```python
from build123d import *

# Parameters (mm, degrees)
SKETCH1_W             = 15
SKETCH1_H             = 15
SKETCH1_R             = 2.6
BOSS_EXTRUDE1_DEPTH   = 6
BOSS_EXTRUDE1_2_DEPTH = 6
BOSS_EXTRUDE1_3_DEPTH = 6
BOSS_EXTRUDE1_4_DEPTH = 6
BOSS_EXTRUDE2_DEPTH   = 64
SKETCH2_R             = 3.05
CUT_EXTRUDE1_DEPTH    = 8
SKETCH3_W             = 15
SKETCH3_H             = 15
SKETCH3_R             = 4.5
BOSS_EXTRUDE3_DEPTH   = 4
CHAMFER1_SIZE         = 0.8
SKETCH4_W             = 200
SKETCH4_H             = 8
BOSS_EXTRUDE4_DEPTH   = 15.5
SKETCH5_W             = 200
SKETCH5_H             = 3
BOSS_EXTRUDE5_DEPTH   = 6
FILLET3_R             = 7.5
FILLET4_R             = 1.5


# Some blends are built 0.0001 mm under size
with BuildPart() as part:
    # Sketch1 → Boss-Extrude1 (new body)
    with BuildSketch(Plane.XY):
        with Locations((-25, 15)):
            Rectangle(SKETCH1_W, SKETCH1_H)
        with Locations((-25, 15)):
            Circle(SKETCH1_R, mode=Mode.SUBTRACT)
    extrude(amount=BOSS_EXTRUDE1_DEPTH)



with BuildPart() as body_2:
    # Sketch1 → Boss-Extrude1 2 (new body)
    with BuildSketch(Plane.XY):
        with Locations((25, 15)):
            Rectangle(SKETCH1_W, SKETCH1_H)
        with Locations((25, 15)):
            Circle(SKETCH1_R, mode=Mode.SUBTRACT)
    extrude(amount=BOSS_EXTRUDE1_2_DEPTH)


with BuildPart() as body_3:
    # Sketch1 → Boss-Extrude1 3 (new body)
    with BuildSketch(Plane.XY):
        with Locations((-75, 15)):
            Rectangle(SKETCH1_W, SKETCH1_H)
        with Locations((-75, 15)):
            Circle(SKETCH1_R, mode=Mode.SUBTRACT)
    extrude(amount=BOSS_EXTRUDE1_3_DEPTH)


with BuildPart() as body_4:
    # Sketch1 → Boss-Extrude1 4 (new body)
    with BuildSketch(Plane.XY):
        with Locations((75, 15)):
            Rectangle(SKETCH1_W, SKETCH1_H)
        with Locations((75, 15)):
            Circle(SKETCH1_R, mode=Mode.SUBTRACT)
    extrude(amount=BOSS_EXTRUDE1_4_DEPTH)


with BuildPart() as part_1:
    add(part.part)

    add(body_2.part)  # Boss-Extrude2 merges body 2

    add(body_3.part)  # Boss-Extrude2 merges body 3
    # Sketch1<4> → Boss-Extrude2 (add)
    with BuildSketch(Plane.XY):
        Polygon((-100, 7.5), (-100, -7.5), (100, -7.5), (100, 7.5), (82.5, 7.5), (67.5, 7.5), (32.5, 7.5), (17.5, 7.5), (-17.5, 7.5), (-32.5, 7.5), (-67.5, 7.5), (-82.5, 7.5), align=None)
    extrude(amount=BOSS_EXTRUDE2_DEPTH)

    # Sketch2 → Cut-Extrude1 (cut)
    with BuildSketch(Plane.XY.offset(64)):
        Circle(SKETCH2_R)
    extrude(amount=-CUT_EXTRUDE1_DEPTH, mode=Mode.SUBTRACT)


    add(body_4.part)  # Boss-Extrude3 merges body 4
    # Sketch3 → Boss-Extrude3 (add)
    # profile 1 of 4: a face of its own
    with BuildSketch(Plane.XY.offset(6)):
        with Locations((75, 15)):
            Rectangle(SKETCH3_W, SKETCH3_H)
        with Locations((75, 15)):
            Circle(SKETCH3_R, mode=Mode.SUBTRACT)
    # profile 2 of 4: a face of its own
    with BuildSketch(Plane.XY.offset(6)):
        with Locations((25, 15)):
            Rectangle(SKETCH3_W, SKETCH3_H)
        with Locations((25, 15)):
            Circle(SKETCH3_R, mode=Mode.SUBTRACT)
    # profile 3 of 4: a face of its own
    with BuildSketch(Plane.XY.offset(6)):
        with Locations((-25, 15)):
            Rectangle(SKETCH3_W, SKETCH3_H)
        with Locations((-25, 15)):
            Circle(SKETCH3_R, mode=Mode.SUBTRACT)
    # profile 4 of 4: a face of its own
    with BuildSketch(Plane.XY.offset(6)):
        with Locations((-75, 15)):
            Rectangle(SKETCH3_W, SKETCH3_H)
        with Locations((-75, 15)):
            Circle(SKETCH3_R, mode=Mode.SUBTRACT)
    extrude(amount=BOSS_EXTRUDE3_DEPTH)

    # Chamfer1
    chamfer1_edges = [part_1.edges().sort_by_distance(p)[0] for p in [
        (-3.05, 0, 64),
    ]]
    chamfer(chamfer1_edges, length=CHAMFER1_SIZE)

    # Sketch4 → Boss-Extrude4 (add)
    with BuildSketch(Plane(origin=(0, 7.5, 0), x_dir=(1, 0, 0), z_dir=(0, 1, 0))):
        with Locations((0, -60)):
            Rectangle(SKETCH4_W, SKETCH4_H)
    extrude(amount=BOSS_EXTRUDE4_DEPTH)

    # Sketch5 → Boss-Extrude5 (add)
    with BuildSketch(Plane.XY.offset(64)):
        with Locations((0, 21.5)):
            Rectangle(SKETCH5_W, SKETCH5_H)
    extrude(amount=BOSS_EXTRUDE5_DEPTH)

    # Fillet3
    # the kernel refuses this fillet: 7.5 mm, written as the material it adds along each edge
    with BuildSketch(Plane(origin=(-82.5, 7.5, 10), x_dir=(0, 1, 0), z_dir=(1, 0, 0))) as fillet3_piece_1_section:
        with BuildLine():
            CenterArc((FILLET3_R, FILLET3_R), FILLET3_R, 180, 90)
            Line((0, FILLET3_R), (0, 0))
            Line((0, 0), (FILLET3_R, 0))
        make_face()
    fillet3_piece_1 = extrude(amount=15, mode=Mode.PRIVATE)
    fillet3_piece_1 = fillet3_piece_1 - Plane(origin=(-75, 15, 10), x_dir=(1, 0, 0), z_dir=(0, 0, -1)) * Cylinder(4.5, 60, mode=Mode.PRIVATE)
    add(fillet3_piece_1)
    with BuildSketch(Plane(origin=(-32.5, 7.5, 10), x_dir=(0, 1, 0), z_dir=(1, 0, 0))) as fillet3_piece_2_section:
        with BuildLine():
            CenterArc((FILLET3_R, FILLET3_R), FILLET3_R, 180, 90)
            Line((0, FILLET3_R), (0, 0))
            Line((0, 0), (FILLET3_R, 0))
        make_face()
    fillet3_piece_2 = extrude(amount=15, mode=Mode.PRIVATE)
    fillet3_piece_2 = fillet3_piece_2 - Plane(origin=(-25, 15, 10), x_dir=(1, 0, 0), z_dir=(0, 0, -1)) * Cylinder(4.5, 61, mode=Mode.PRIVATE)
    add(fillet3_piece_2)
    with BuildSketch(Plane(origin=(17.5, 7.5, 10), x_dir=(0, 1, 0), z_dir=(1, 0, 0))) as fillet3_piece_3_section:
        with BuildLine():
            CenterArc((FILLET3_R, FILLET3_R), FILLET3_R, 180, 90)
            Line((0, FILLET3_R), (0, 0))
            Line((0, 0), (FILLET3_R, 0))
        make_face()
    fillet3_piece_3 = extrude(amount=15, mode=Mode.PRIVATE)
    fillet3_piece_3 = fillet3_piece_3 - Plane(origin=(25, 15, 10), x_dir=(1, 0, 0), z_dir=(0, 0, -1)) * Cylinder(4.5, 61, mode=Mode.PRIVATE)
    add(fillet3_piece_3)
    with BuildSketch(Plane(origin=(67.5, 7.5, 10), x_dir=(0, 1, 0), z_dir=(1, 0, 0))) as fillet3_piece_4_section:
        with BuildLine():
            CenterArc((FILLET3_R, FILLET3_R), FILLET3_R, 180, 90)
            Line((0, FILLET3_R), (0, 0))
            Line((0, 0), (FILLET3_R, 0))
        make_face()
    fillet3_piece_4 = extrude(amount=15, mode=Mode.PRIVATE)
    fillet3_piece_4 = fillet3_piece_4 - Plane(origin=(75, 15, 10), x_dir=(1, 0, 0), z_dir=(0, 0, -1)) * Cylinder(4.5, 60, mode=Mode.PRIVATE)
    add(fillet3_piece_4)
    with BuildSketch(Plane(origin=(100, 7.5, 56), x_dir=(0, 0, -1), z_dir=(-1, 0, 0))) as fillet3_piece_5:
        with BuildLine():
            CenterArc((FILLET3_R, -FILLET3_R), FILLET3_R, 90, 90)
            Line((0, -FILLET3_R), (0, 0))
            Line((0, 0), (FILLET3_R, 0))
        make_face()
    extrude(amount=200)
    # the kernel refuses this fillet: 7.5 mm, written as the material it takes off along each edge
    with BuildSketch(Plane(origin=(100, -7.5, -18.75), x_dir=(-1, 0, 0), z_dir=(0, 0, 1))) as fillet3_2_piece_1:
        with BuildLine():
            CenterArc((FILLET3_R, -FILLET3_R), FILLET3_R, 90, 90)
            Line((0, -FILLET3_R), (0, 0))
            Line((0, 0), (FILLET3_R, 0))
        make_face()
    extrude(amount=101.5, mode=Mode.SUBTRACT)
    with BuildSketch(Plane(origin=(-100, -7.5, -18.75), x_dir=(1, 0, 0), z_dir=(0, 0, 1))) as fillet3_2_piece_2:
        with BuildLine():
            CenterArc((FILLET3_R, FILLET3_R), FILLET3_R, 180, 90)
            Line((0, FILLET3_R), (0, 0))
            Line((0, 0), (FILLET3_R, 0))
        make_face()
    extrude(amount=101.5, mode=Mode.SUBTRACT)
    with BuildSketch(Plane(origin=(67.5, 22.5, 28.75), x_dir=(0, -1, 0), z_dir=(0, 0, -1)), Plane(origin=(-82.5, 22.5, 28.75), x_dir=(0, -1, 0), z_dir=(0, 0, -1)), Plane(origin=(17.5, 22.5, 28.75), x_dir=(0, -1, 0), z_dir=(0, 0, -1)), Plane(origin=(-32.5, 22.5, 28.75), x_dir=(0, -1, 0), z_dir=(0, 0, -1))) as fillet3_2_piece_3:
        with BuildLine():
            CenterArc((FILLET3_R, -FILLET3_R), FILLET3_R, 90, 90)
            Line((0, -FILLET3_R), (0, 0))
            Line((0, 0), (FILLET3_R, 0))
        make_face()
    extrude(amount=47.5, mode=Mode.SUBTRACT)
    with BuildSketch(Plane(origin=(-67.5, 22.5, -18.75), x_dir=(-1, 0, 0), z_dir=(0, 0, 1)), Plane(origin=(-17.5, 22.5, -18.75), x_dir=(-1, 0, 0), z_dir=(0, 0, 1)), Plane(origin=(32.5, 22.5, -18.75), x_dir=(-1, 0, 0), z_dir=(0, 0, 1)), Plane(origin=(82.5, 22.5, -18.75), x_dir=(-1, 0, 0), z_dir=(0, 0, 1))) as fillet3_2_piece_4:
        with BuildLine():
            CenterArc((FILLET3_R, FILLET3_R), FILLET3_R, 180, 90)
            Line((0, FILLET3_R), (0, 0))
            Line((0, 0), (FILLET3_R, 0))
        make_face()
    extrude(amount=47.5, mode=Mode.SUBTRACT)
    with BuildSketch(Plane(origin=(118.75, 23, 56), x_dir=(0, -1, 0), z_dir=(-1, 0, 0))) as fillet3_2_piece_5:
        with BuildLine():
            CenterArc((FILLET3_R, FILLET3_R), FILLET3_R, 180, 90)
            Line((0, FILLET3_R), (0, 0))
            Line((0, 0), (FILLET3_R, 0))
        make_face()
    extrude(amount=237.5, mode=Mode.SUBTRACT)
    # the kernel refuses this fillet: 7.5 mm, written as the material it takes off along each edge
    with BuildSketch(Plane(origin=(-100, 7.5, -18.75), x_dir=(0, -1, 0), z_dir=(0, 0, 1)), Plane(origin=(100, 7.5, -18.75), x_dir=(-1, 0, 0), z_dir=(0, 0, 1))) as fillet3_3_piece_1:
        with BuildLine():
            CenterArc((FILLET3_R, FILLET3_R), FILLET3_R, 180, 90)
            Line((0, FILLET3_R), (0, 0))
            Line((0, 0), (FILLET3_R, 0))
        make_face()
    extrude(amount=67.25, mode=Mode.SUBTRACT)
    with BuildSketch(Plane(origin=(100, 15, 56), x_dir=(-1, 0, 0), z_dir=(0, 1, 0)), Plane(origin=(-100, 15, 56), x_dir=(0, 0, 1), z_dir=(0, 1, 0))) as fillet3_3_piece_2:
        with BuildLine():
            CenterArc((FILLET3_R, FILLET3_R), FILLET3_R, 180, 90)
            Line((0, FILLET3_R), (0, 0))
            Line((0, 0), (FILLET3_R, 0))
        make_face()
    extrude(amount=19.25, mode=Mode.SUBTRACT)
    with BuildSketch(Plane(origin=(-100, 15, 48.5), x_dir=(0, -1, 0), z_dir=(0, 0, -1))) as fillet3_3_piece_3:
        with BuildLine():
            CenterArc((7.5 + FILLET3_R, -FILLET3_R), FILLET3_R, 90, 90)
            Line((7.5, -FILLET3_R), (7.5, 0))
            Line((7.5, 0), (7.5 + FILLET3_R, 0))
        make_face()
    revolve(axis=Axis((-100, 15, 48.5), (-1, 0, 0)), revolution_arc=90, mode=Mode.SUBTRACT)
    with BuildSketch(Plane(origin=(100, 15, 48.5), x_dir=(0, -1, 0), z_dir=(0, 0, -1))) as fillet3_3_piece_4:
        with BuildLine():
            CenterArc((7.5 + FILLET3_R, FILLET3_R), FILLET3_R, 180, 90)
            Line((7.5 + FILLET3_R, 0), (7.5, 0))
            Line((7.5, 0), (7.5, FILLET3_R))
        make_face()
    revolve(axis=Axis((100, 15, 48.5), (-1, 0, 0)), revolution_arc=90, mode=Mode.SUBTRACT)

    # Fillet4
    fillet4_edges = [part_1.edges().sort_by_distance(p)[0] for p in [
        (-97.803300859, 20.803300859, 58.196699141),
        (97.803300859, 20.803300859, 58.196699141),
        (-100, 20, 67),
        (-100, 23, 66.75),
        (100, 23, 66.75),
        (100, 20, 67),
    ]]
    fillet(fillet4_edges, radius=FILLET4_R - 0.0001)  # a hair under: the kernel refuses the full size


solid = part_1.part
```
Geometry: final body of the model. Coordinates: model frame, mm. A direction names the side the tool comes from. Round coordinates to 2 decimals unless told otherwise and drop trailing zeros. Order: outer loops, then holes, each group sorted by start corner. A loop starts at its lowest first (then second) coordinate and runs counter-clockwise, first axis right, second up. Notation, with made-up numbers: (68, 52) -> (108, 52) arc R34 cw to (108, 85) -> close; hole circle Ø11 at (9, -35.75). An arc over 180 degrees is marked (long way). Use one line per item in the form item = value.
(1) First-contact query: pin 1 Ø10 at (x, z) = (54, 10.5) entering from +Y; pin 2 Ø6 at (y, z) = (12, 9.5) entering from +X; pin 3 Ø2 at (y, z) = (5, 50) entering from -X. Flat tips, straight axial feed; report the tip coordinate or a pass-through.
Results list:
pin_1 = 7.5
pin_2 = 82.5
pin_3 = -98.91
(2) Section A-A on x = -75. Return loops of the section in (y, z).
Results list:
outline = (-7.5, 0) -> (12.4, 0) -> (12.4, 6) -> (10.5, 6) -> (10.5, 11.5) arc R7.5 cw to (7.5, 17.5) -> (7.5, 48.5) arc R7.5 cw to (15, 56) -> (15.5, 56) arc R7.5 ccw to (23, 63.5) -> (23, 70) -> (20, 70) -> (20, 64) -> (-7.5, 64) -> close; (17.6, 0) -> (22.5, 0) -> (22.5, 10) -> (19.5, 10) -> (19.5, 6) -> (17.6, 6) -> close
(3) Ray query, probe 1 along Y at (x, z) = (-55.5, 47); probe 2 along Y at (x, z) = (75, 8.85); probe 3 along Y at (x, z) = (25, 3). Return the intervals inside material, ascending. Write a range as [from, to].
Results list:
probe_1 = [-7.5, 7.5]
probe_2 = [-7.5, 10.5], [19.5, 22.5]
probe_3 = [-7.5, 12.4], [17.6, 22.5]
(4) Draft query along X for faces 1 (the face through (-100, 0, 32)), 2 (the face through (77, 13, 6)), 3 (the face through (-25, 20, 10)). Return one class per face: pulls with the +X half, pulls with the -X half, needs draft (parallel to the pull), parting line crosses it, or undercut.
Results list:
face_1 = pulls with the -X half
face_2 = undercut
face_3 = needs draft
(5) Section C-C on z = 40. Return loops of the section in (x, y), and give its area (3 significant figures).
Results list:
outline = (-92.5, -7.5) -> (92.5, -7.5) arc R7.5 ccw to (92.5, 7.5) -> (-92.5, 7.5) arc R7.5 ccw to start
area = 2,950 mm^2
(6) Access query for faces 4 (the face through (74.84, 22.5, 5.07)), 5 (the face through (-77.6, 15.1, 3)), 6 (the face through (-98.596, 17.482, 59.131)), 7 (the face through (98.691, 17.482, 59.266)), 8 (the face through (-25.98, 10.61, 8.1)). Directions: +Z, -Z, +X, -X, +Y, -Y. A direction counts if a zero-diameter tool reaches every point of the face in a straight line with its end or side. Return the directions, or none.
Results list:
face_4 = -Z, +Y
face_5 = -Z
face_6 = -Z, -X, +Y
face_7 = -Z, +X, +Y
face_8 = none
(7) Section B-B on x = -7. Return loops of the section in (y, z).
Results list:
outline = (-7.5, 0) -> (7.5, 0) -> (7.5, 48.5) arc R7.5 cw to (15, 56) -> (15.5, 56) arc R7.5 ccw to (23, 63.5) -> (23, 70) -> (20, 70) -> (20, 64) -> (-7.5, 64) -> close
